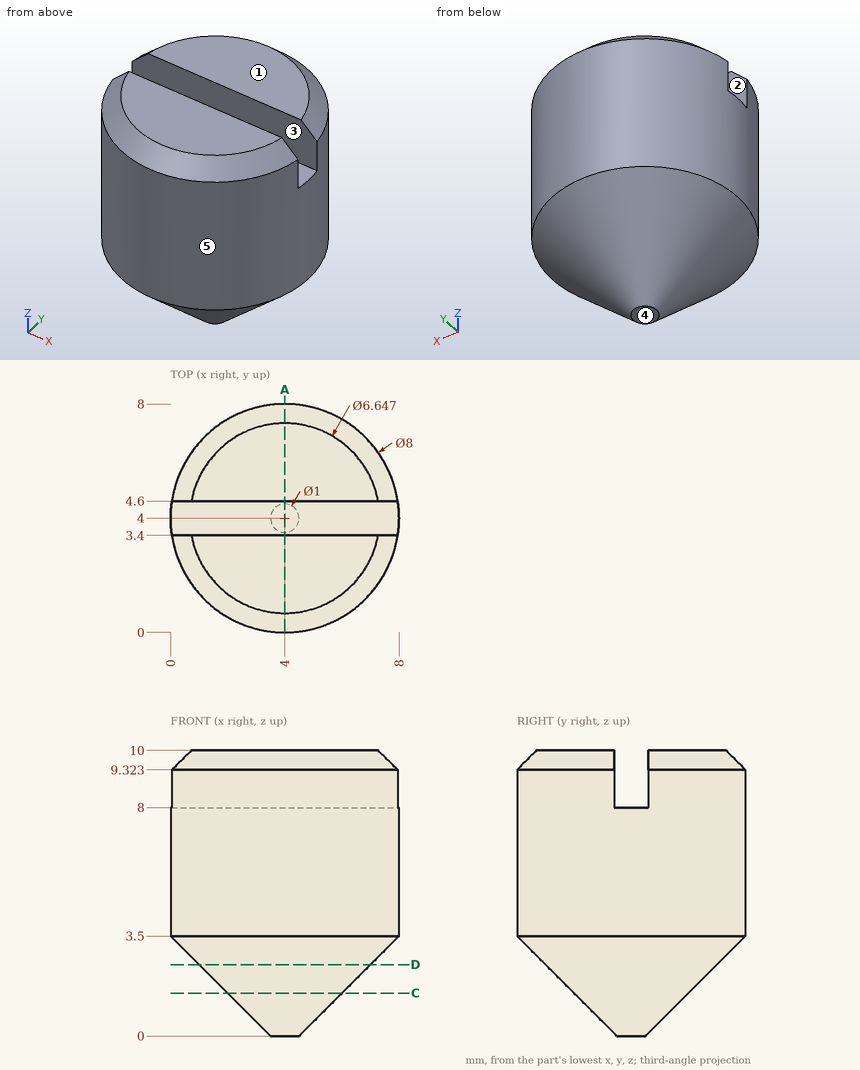
Source: three-view drawing plus pictorial views. Frame: mm from the lowest corner of the part. A direction names the side the tool comes from. Round coordinates to 2 decimals unless told otherwise and drop trailing zeros. Write each loop counter-clockwise with the first axis right and the second up, starting at its lowest first coordinate (ties: lowest second). Pieces come first, ordered by that corner, then holes. Notation, with made-up numbers: M 48.25,43 L 92.25,43 A12 ccw 92.25,55 Z; hole C 10.5,40.25 d2. An arc over 180 degrees is marked long. Write each question's results on one line, items separated by ' | '.
Q1. Access query for the marked faces 1 and 2. Directions: +Z, -Z, +X, -X, +Y, -Y. A direction counts if a zero-diameter tool reaches every point of the face in a straight line with its end or side. Return the directions, or none.
Results:
face 1: +Z, +X, -X, +Y, -Y | face 2: +Z, +X, -X
Q2. Draft query along Y for the marked faces 3, 4 and 5. Return one class per face: released by +Y, released by -Y, zero draft, split by the parting line, or undercut.
Results:
face 3: undercut | face 4: zero draft | face 5: split by the parting line
Q3. Section query C-C (z = 1.5). Return loops of the section in (x, y).
Results:
outline: C 4,4 d4
Q4. Section query A-A (x = 4). Return loops of the section in (y, z), and give its area (3 significant figures).
Results:
outline: M 0,3.5 L 3.5,0 L 4.5,0 L 8,3.5 L 8,9.32 L 7.32,10 L 4.6,10 L 4.6,8 L 3.4,8 L 3.4,10 L 0.68,10 L 0,9.32 Z | area: 64.9 mm^2
Q5. Section query D-D (z = 2.5). Return loops of the section in (x, y), and give its area (3 significant figures).
Results:
outline: C 4,4 d6 | area: 28.3 mm^2
Q6. Pin query (flat end, axial travel): P1, Ø1, axis at x = 6, y = 5, coming from the -Z side (1 decimal). Return the tip coordinate at first contact, or that it passes through.
Results:
P1: stops at z = 1.2
Q7. Line query: line 1 along Y through (x, z) = (4, 8.5); line 2 along Z through (x, y) = (3, 1.25) (1 decimal); line 3 along Z through (x, y) = (4.75, 4.5). Output: solid intervals per line, ascending.
Results:
line 1: y = 0 to 3.4, 4.6 to 8 | line 2: z = 2.4 to 10 | line 3: z = 0.4 to 8
